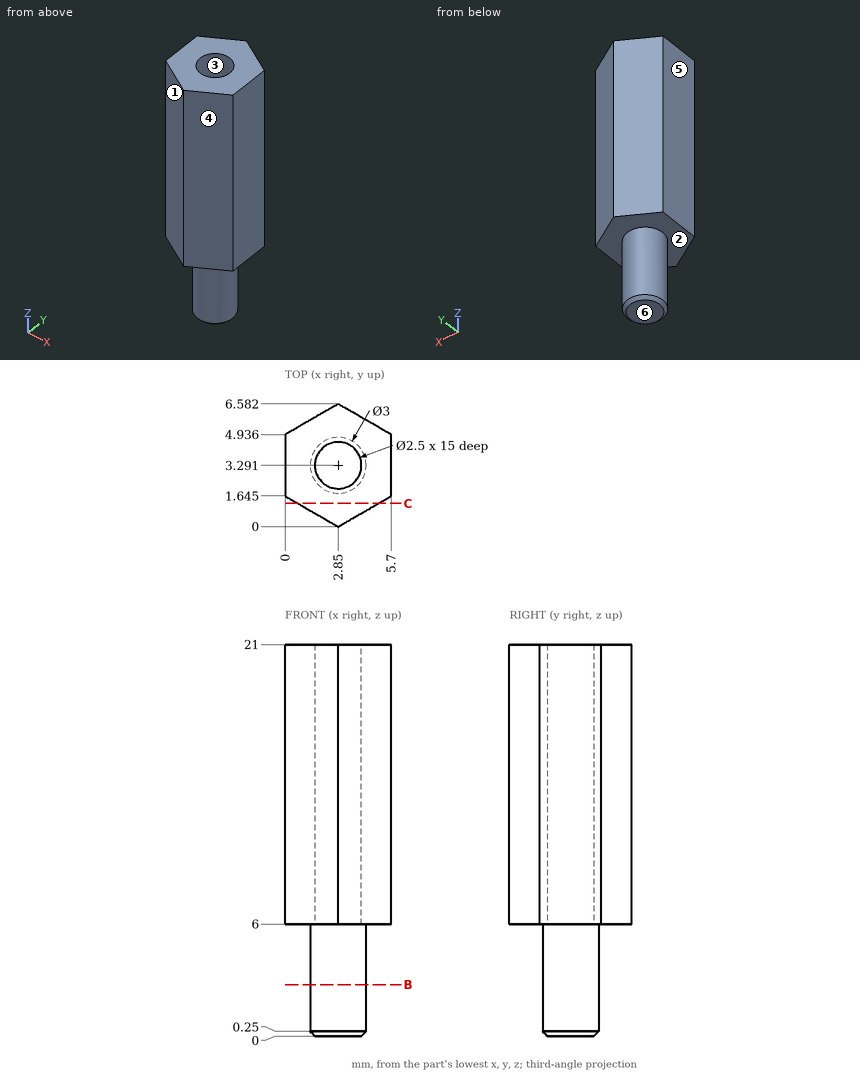
Can you work these out from the drawing? Everything is in mm from the part's minimum corner. A direction names the side the tool comes from. Round coordinates to 2 decimals unless told otherwise and drop trailing zeros. Loops run counter-clockwise (first coordinate to the right, second up) from the corner with the lowest first, then second, coordinate; pieces in that order, holes last. Notation, with made-up numbers: (21.5, 42) - (31.5, 42) arc R19 ccw to (31.5, 55) - close; hole circle Ø8 at (-11, -13). An arc over 180 degrees is marked (long way). One line per question, with ' | ' between items. Start each with the question number.
Q1. Please list where these lines run through material, in increasing order: line 1 (Z direction, x = 2.4, y = 2.5); line 2 (X direction, y = 3.25, z = 1.5); line 3 (Z direction, x = 1.65, y = 1.25). Write a range as [from, to].
Q2. For the marked faces 1 and 2, which set-ups out of +Z, -Z, +X, -X, +Y, -Y let a thin tool reach every point of the face, with its end or its side?
Q3. I want a section at C-C (y = 1.25). Write out the boundary of the cut face in (x, z) (1 decimal).
Q4. Will this pin go through, and if not, where does the flat tip stop? pin 1 (2 mm diameter, centred on x = 2.85, y = 3.29, fed in from +Z).
Q5. I want a section at B-B (z = 2.75). Write out the boundary of the cut face in (x, y).
Q6. We'd pull the mould along X, two halves only. Please class the marked faces 3, 4, 5 and 6: +X half, -X half, draft (parallel to the pull), parting line (faces both ways), or undercut.
Response values:
1) line 1: z = [0, 6] | line 2: x = [1.35, 4.35] | line 3: z = [6, 21]
2) face 1: +Z, -Z, -X, -Y | face 2: -Z
3) outline: (0.7, 6) - (5, 6) - (5, 21) - (0.7, 21) - close
4) pin 1: stops at z = 6
5) outline: circle Ø3 at (2.85, 3.29)
6) face 3: undercut | face 4: +X half | face 5: -X half | face 6: draft
